from build123d import *

# Parameters (mm, degrees)
CROQUIS1_R                               = 24.6
CROQUIS1_R_2                             = 19.6
SALIENTE_EXTRUIR1_DEPTH                  = 11
CROQUIS2_W                               = 22
CROQUIS2_H                               = 23
CROQUIS2_R                               = 8.5
SALIENTE_EXTRUIR2_DEPTH                  = 25
SALIENTE_EXTRUIR2_DIRECTION_2_REACH      = 58.096
SALIENTE_EXTRUIR2_DIRECTION_2_END_RADIUS = 24.6
CROQUIS3_R                               = 2
CORTAR_EXTRUIR1_DEPTH                    = 47.5
CROQUIS4_R                               = 2
CORTAR_EXTRUIR2_DEPTH                    = 95
REDONDEO1_R                              = 80


with BuildPart() as part:
    # Croquis1 → Saliente-Extruir1 (new, symmetric)
    with BuildSketch(Plane.XY):
        Circle(CROQUIS1_R)
        Circle(CROQUIS1_R_2, mode=Mode.SUBTRACT)
    extrude(amount=SALIENTE_EXTRUIR1_DEPTH, both=True)

    # Croquis2 → Saliente-Extruir2 (add)
    with BuildSketch(Plane(origin=(24.6, 0, 0), x_dir=(0, 0, -1), z_dir=(1, 0, 0))):
        Rectangle(CROQUIS2_W, CROQUIS2_H)
        Circle(CROQUIS2_R, mode=Mode.SUBTRACT)
    extrude(amount=SALIENTE_EXTRUIR2_DEPTH)

    # Saliente-Extruir2 direction 2: up to this cylinder (the profile starts outside it)
    saliente_extruir2_direction_2_end = Plane(origin=(0, 0, 0), z_dir=(0, 0, -1)) * Cylinder(SALIENTE_EXTRUIR2_DIRECTION_2_END_RADIUS, 166.392, mode=Mode.PRIVATE)
    # Croquis2 → Saliente-Extruir2 direction 2 (add, up to the surface)
    with BuildSketch(Plane(origin=(24.6, 0, 0), x_dir=(0, 0, -1), z_dir=(1, 0, 0)), mode=Mode.PRIVATE) as saliente_extruir2_direction_2_sk1:
        Rectangle(CROQUIS2_W, CROQUIS2_H)
        Circle(CROQUIS2_R, mode=Mode.SUBTRACT)
    saliente_extruir2_direction_2_tool1 = extrude(saliente_extruir2_direction_2_sk1.sketch, amount=-SALIENTE_EXTRUIR2_DIRECTION_2_REACH, mode=Mode.PRIVATE) - saliente_extruir2_direction_2_end
    add(saliente_extruir2_direction_2_tool1.solids().sort_by_distance((24.6, -11.181723, 0))[0])
    add(saliente_extruir2_direction_2_tool1.solids().sort_by_distance((24.6, -11.181723, 0))[1])

    # Croquis3 → Cortar-Extruir1 (cut, symmetric)
    with BuildSketch(Plane(origin=(0, 0, 0), x_dir=(1, 0, 0), z_dir=(0, 1, 0))):
        with Locations(Location((0, 0, 0), (0, 0, 270))):
            Circle(CROQUIS3_R)
    extrude(amount=CORTAR_EXTRUIR1_DEPTH, both=True, mode=Mode.SUBTRACT)

    # Croquis4 → Cortar-Extruir2 (cut)
    with BuildSketch(Plane(origin=(0, 0, 0), x_dir=(0, 0, -1), z_dir=(1, 0, 0))):
        Circle(CROQUIS4_R)
    extrude(amount=-CORTAR_EXTRUIR2_DEPTH, mode=Mode.SUBTRACT)

    # Redondeo1
    # the kernel refuses this fillet: 80 mm, written as the material it adds along each edge
    with BuildSketch(Plane(origin=(21.74649397, 11.5, 11), x_dir=(-0.7001557683573276, 0.713990126007328, 0), z_dir=(0, 0, -1))) as redondeo1_piece_1:
        with BuildLine():
            CenterArc((36.84325364, 76.678287175), REDONDEO1_R, 225.225924333, 28.205393766)
            Line((-19.501792916, 19.88712828), (-20.628693847, 18.751305102))
            ThreePointArc((-20.628693847, 18.751305102), (-10.893280659, 8.823314911), (-1.142384202, -1.120249229))
            Line((-1.142384202, -1.120249229), (0.456263203, -1.533565743))
            ThreePointArc((0.456263203, -1.533565743), (7.015046746, -0.578573306), (13.573830289, -1.533565743))
            Line((13.573830289, -1.533565743), (14.030093492, 0))
        make_face()
    extrude(amount=22)
    with BuildSketch(Plane(origin=(21.74649397, -11.5, 11), x_dir=(-0.7001557683573284, -0.7139901260073274, 0), z_dir=(0, 0, -1))) as redondeo1_piece_2:
        with BuildLine():
            CenterArc((36.84325364, -76.678287175), REDONDEO1_R, 106.568681901, 28.205393766)
            Line((-19.501792916, -19.88712828), (-20.628693847, -18.751305102))
            ThreePointArc((-20.628693847, -18.751305102), (-10.893280659, -8.823314911), (-1.142384202, 1.120249229))
            Line((-1.142384202, 1.120249229), (0.456263203, 1.533565743))
            ThreePointArc((0.456263203, 1.533565743), (7.015046746, 0.578573306), (13.573830289, 1.533565743))
            Line((13.573830289, 1.533565743), (14.030093492, 0))
        make_face()
    extrude(amount=22)


solid = part.part
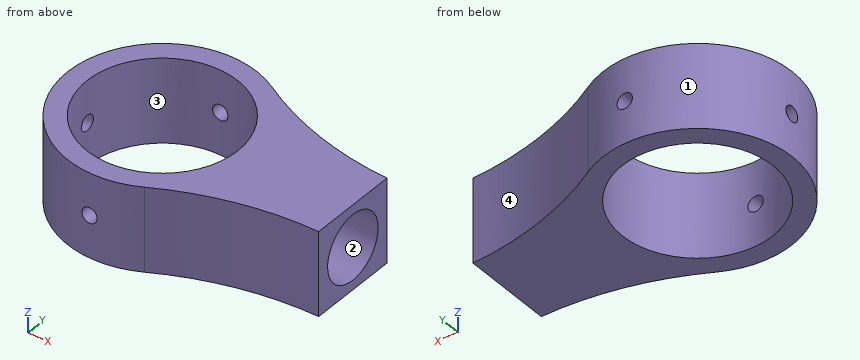
The listing builds one solid part. Answer for the finished solid, in the listing's coordinates (mm). Face numbers are marked on the shaded views. Round coordinates to 2 decimals unless told otherwise and drop trailing zeros. Order: outer loops, then holes, each group sorted by start corner. A loop starts at its lowest first (then second) coordinate and runs counter-clockwise, first axis right, second up. Notation, with made-up numbers: (13.5, 6.5) - (60.5, 6.5) arc R10 cw to (60.5, 25.5) - close; hole circle Ø3 at (70.25, 87). An arc over 180 degrees is marked (long way). Write item = value, one per line. Start each with the question number.
1) Section A-A, the plane y = 0 is taken. Write down the section's boundary in (x, z).
2) Section C-C, the plane z = 0.25 is taken. Write down the section's boundary in (x, y), plus the area to 3 significant figures.
3) Given pin 1 (1 mm diameter, centred on x = 1, z = 1.5, fed in from -Y); pin 2 (4 mm diameter, centred on y = 4, z = -3, fed in from -X); pin 3 (6 mm diameter, centred on x = 5.5, z = -1.5, fed in from -Y), each flat-ended and moving along its own axis, determine where each tip first touches the part or whether it passes through.
4) For a pull along X with two mould halves and no side action, classify the marked faces 1, 2, 3 and 4 as released by +X, released by -X, zero draft, split by the parting line, or undercut.
5) Section D-D, the plane x = 10 is taken. Write down the section's boundary in (y, z).
6) Section B-B, the plane x = 0 is taken. Write down the section's boundary in (y, z).
7) Straight lines are drawn through the part: L1, parallel to Y at x = -0.5, z = -9; L2, parallel to Z at x = 43, y = 0; L3, parallel to Z at x = 0, y = -22. For each, find the intervals that lie inside material, in ascending order.
Results list:
q1.outline = (-24.6, -11) - (-19.6, -11) - (-19.6, -2) - (-24.6, -2) - close; (-24.6, 2) - (-19.6, 2) - (-19.6, 11) - (-24.6, 11) - close; (19.6, -11) - (49.6, -11) - (49.6, -8.5) - (24.6, -8.5) - (24.6, 8.5) - (49.6, 8.5) - (49.6, 11) - (19.6, 11) - close
q2.outline = (-24.52, -1.98) arc R24.6 ccw to (-1.98, -24.52) - (-1.98, -19.5) arc R19.6 cw to (-19.5, -1.98) - close; (-24.52, 1.98) - (-19.5, 1.98) arc R19.6 cw to (-1.98, 19.5) - (-1.98, 24.52) arc R24.6 ccw to start; (1.98, -24.52) arc R24.6 ccw to (11.92, -21.52) arc R80 cw to (49.6, -11.5) - (49.6, -8.5) - (23.09, -8.5) arc R24.6 ccw to (23.09, 8.5) - (49.6, 8.5) - (49.6, 11.5) arc R80 cw to (11.92, 21.52) arc R24.6 ccw to (1.98, 24.52) - (1.98, 19.5) arc R19.6 cw to (1.98, -19.5) - close
q2.area = 932 mm^2
q3.pin_1 = -24.59
q3.pin_2 = -24.52
q3.pin_3 = -24.47
q4.face_1 = split by the parting line
q4.face_2 = zero draft
q4.face_3 = undercut
q4.face_4 = released by +X
q5.outline = (-22.48, -11) - (-16.86, -11) - (-16.86, 11) - (-22.48, 11) - close; (16.86, -11) - (22.48, -11) - (22.48, 11) - (16.86, 11) - close
q6.outline = (-24.6, -11) - (-19.6, -11) - (-19.6, -2) - (-24.6, -2) - close; (-24.6, 2) - (-19.6, 2) - (-19.6, 11) - (-24.6, 11) - close; (19.6, -11) - (24.6, -11) - (24.6, -2) - (19.6, -2) - close; (19.6, 2) - (24.6, 2) - (24.6, 11) - (19.6, 11) - close
q7.L1 = -24.59 to -19.59, 19.59 to 24.59
q7.L2 = -11 to -8.5, 8.5 to 11
q7.L3 = -11 to -2, 2 to 11
